Verification items for the finished model (mm, model axes). Face numbers are marked on the shaded views. Give positions to 0.01 mm unless a question says otherwise; leave off trailing zeros. Loops run counter-clockwise (first coordinate to the right, second up) from the corner with the lowest first, then second, coordinate; pieces in that order, holes last. Notation, with made-up numbers: M 42.5,81 L 47.5,81 A20 cw 47.5,96 Z; hole C 39,7 d9. An arc over 180 degrees is marked long. Put each result on its own line as item: value. Start each with the question number.
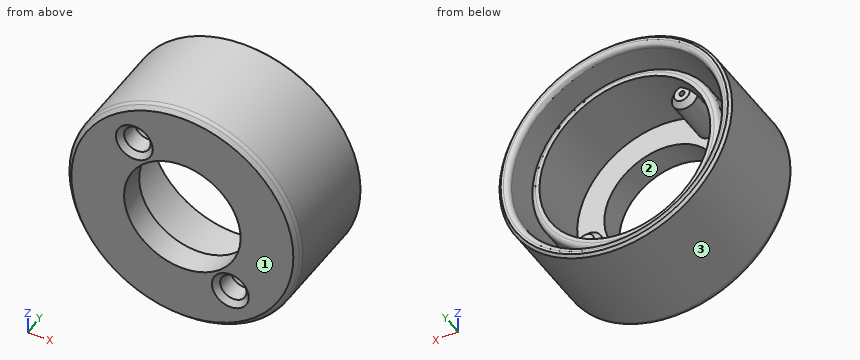
from build123d import *
from OCP.BRepFilletAPI import BRepFilletAPI_MakeChamfer

# Parameters (mm, degrees)
CROQUIS1_R              = 22.05
CROQUIS1_R_2            = 20.05
SALIENTE_EXTRUIR1_DEPTH = 16
CROQUIS1_4_R            = 17.95
CROQUIS1_4_R_2          = 16.2
SALIENTE_EXTRUIR2_DEPTH = 12.5
SALIENTE_EXTRUIR4_START = -5
CROQUIS1_6_R            = 22.05
CROQUIS1_6_R_2          = 20.05
CROQUIS1_6_R_3          = 17.95
CROQUIS1_6_R_4          = 16.2
SALIENTE_EXTRUIR4_DEPTH = 5
CORTAR_EXTRUIR1_REACH   = 39.595
CROQUIS4_R              = 11.05
CROQUIS4_R_2            = 0.5
CROQUIS5_R              = 2.5
CROQUIS5_R_2            = 0.5
CORTAR_EXTRUIR2_DEPTH   = 4.5
CROQUIS6_R              = 2.5
CROQUIS6_R_2            = 0.5
SALIENTE_EXTRUIR5_DEPTH = 10
REDONDEO2_R             = 1
CHAFL_N1_SIZE           = 1
REDONDEO3_R             = 1
CHAFL_N2_SIZE           = 0.5
CHAFL_N3_SIZE           = 2
CHAFL_N3_SIZE_2         = 1.154700538


with BuildPart() as part:
    # Croquis1 → Saliente-Extruir1 (new body)
    with BuildSketch(Plane(origin=(0, 0, 0), x_dir=(1, 0, 0), z_dir=(0, 1, 0))):
        with Locations(Location((0, 0, 0), (0, 0, 270))):
            Circle(CROQUIS1_R)
        with Locations(Location((0, 0, 0), (0, 0, 270))):
            Circle(CROQUIS1_R_2, mode=Mode.SUBTRACT)
    extrude(amount=SALIENTE_EXTRUIR1_DEPTH)



with BuildPart() as body_2:
    # Croquis1<4> → Saliente-Extruir2 (new body)
    with BuildSketch(Plane(origin=(0, 0, 0), x_dir=(1, 0, 0), z_dir=(0, 1, 0))):
        with Locations(Location((0, 0, 0), (0, 0, 270))):
            Circle(CROQUIS1_4_R)
        with Locations(Location((0, 0, 0), (0, 0, 270))):
            Circle(CROQUIS1_4_R_2, mode=Mode.SUBTRACT)
    extrude(amount=SALIENTE_EXTRUIR2_DEPTH)


with BuildPart() as part_1:
    add(part.part)

    add(body_2.part)  # Saliente-Extruir4 merges body 2
    # Croquis1<6> → Saliente-Extruir4 (add)
    # profile 1 of 4: a face of its own
    with BuildSketch(Plane(origin=(0, 0, 0), x_dir=(1, 0, 0), z_dir=(0, 1, 0)).offset(SALIENTE_EXTRUIR4_START)):
        with Locations(Location((0, 0, 0), (0, 0, 270))):
            Circle(CROQUIS1_6_R)
        with Locations(Location((0, 0, 0), (0, 0, 270))):
            Circle(CROQUIS1_6_R_2, mode=Mode.SUBTRACT)
    # profile 2 of 4: a face of its own
    with BuildSketch(Plane(origin=(0, 0, 0), x_dir=(1, 0, 0), z_dir=(0, 1, 0)).offset(SALIENTE_EXTRUIR4_START)):
        with Locations(Location((0, 0, 0), (0, 0, 270))):
            Circle(CROQUIS1_6_R_2)
        with Locations(Location((0, 0, 0), (0, 0, 270))):
            Circle(CROQUIS1_6_R_3, mode=Mode.SUBTRACT)
    # profile 3 of 4: a face of its own
    with BuildSketch(Plane(origin=(0, 0, 0), x_dir=(1, 0, 0), z_dir=(0, 1, 0)).offset(SALIENTE_EXTRUIR4_START)):
        with Locations(Location((0, 0, 0), (0, 0, 270))):
            Circle(CROQUIS1_6_R_3)
        with Locations(Location((0, 0, 0), (0, 0, 270))):
            Circle(CROQUIS1_6_R_4, mode=Mode.SUBTRACT)
    # profile 4 of 4: a face of its own
    with BuildSketch(Plane(origin=(0, 0, 0), x_dir=(1, 0, 0), z_dir=(0, 1, 0)).offset(SALIENTE_EXTRUIR4_START)):
        with Locations(Location((0, 0, 0), (0, 0, 270))):
            Circle(CROQUIS1_6_R_4)
    extrude(amount=SALIENTE_EXTRUIR4_DEPTH)

    # Croquis4 → Cortar-Extruir1 (cut, up to next)
    with BuildSketch(Plane.XZ.offset(5), mode=Mode.PRIVATE) as cortar_extruir1_sk1:
        with Locations(Location((0, 0, 0), (0, 0, 270))):
            Circle(CROQUIS4_R)
    cortar_extruir1_tool1 = extrude(cortar_extruir1_sk1.sketch, amount=-CORTAR_EXTRUIR1_REACH, mode=Mode.PRIVATE) & part_1.part
    # Croquis4 → Cortar-Extruir1 (cut, up to next)
    with BuildSketch(Plane.XZ.offset(5), mode=Mode.PRIVATE) as cortar_extruir1_sk2:
        with Locations(Location((-9.1, 12.1, 0), (0, 0, 270))):
            Circle(CROQUIS4_R_2)
    cortar_extruir1_tool2 = extrude(cortar_extruir1_sk2.sketch, amount=-CORTAR_EXTRUIR1_REACH, mode=Mode.PRIVATE) & part_1.part
    # Croquis4 → Cortar-Extruir1 (cut, up to next)
    with BuildSketch(Plane.XZ.offset(5), mode=Mode.PRIVATE) as cortar_extruir1_sk3:
        with Locations(Location((9.1, -12.1, 0), (0, 0, 270))):
            Circle(CROQUIS4_R_2)
    cortar_extruir1_tool3 = extrude(cortar_extruir1_sk3.sketch, amount=-CORTAR_EXTRUIR1_REACH, mode=Mode.PRIVATE) & part_1.part
    add(cortar_extruir1_tool1.solids().sort_by_distance((0, -5, 0))[0], mode=Mode.SUBTRACT)
    add(cortar_extruir1_tool2.solids().sort_by_distance((-9.1, -5, 12.1))[0], mode=Mode.SUBTRACT)
    add(cortar_extruir1_tool3.solids().sort_by_distance((9.1, -5, -12.1))[0], mode=Mode.SUBTRACT)

    # Croquis5 → Cortar-Extruir2 (cut)
    # profile 1 of 2: a face of its own
    with BuildSketch(Plane.XZ.offset(5)):
        with Locations(Location((-9.1, 12.1, 0), (0, 0, 270))):
            Circle(CROQUIS5_R)
        with Locations(Location((-9.1, 12.1, 0), (0, 0, 270))):
            Circle(CROQUIS5_R_2, mode=Mode.SUBTRACT)
    # profile 2 of 2: a face of its own
    with BuildSketch(Plane.XZ.offset(5)):
        with Locations(Location((9.1, -12.1, 0), (0, 0, 270))):
            Circle(CROQUIS5_R)
        with Locations(Location((9.1, -12.1, 0), (0, 0, 270))):
            Circle(CROQUIS5_R_2, mode=Mode.SUBTRACT)
    extrude(amount=-CORTAR_EXTRUIR2_DEPTH, mode=Mode.SUBTRACT)

    # Croquis6 → Saliente-Extruir5 (add)
    # profile 1 of 2: a face of its own
    with BuildSketch(Plane.XZ.offset(0.5)):
        with Locations(Location((-9.1, 12.1, 0), (0, 0, 270))):
            Circle(CROQUIS6_R)
        with Locations(Location((-9.1, 12.1, 0), (0, 0, 270))):
            Circle(CROQUIS6_R_2, mode=Mode.SUBTRACT)
    # profile 2 of 2: a face of its own
    with BuildSketch(Plane.XZ.offset(0.5)):
        with Locations(Location((9.1, -12.1, 0), (0, 0, 270))):
            Circle(CROQUIS6_R)
        with Locations(Location((9.1, -12.1, 0), (0, 0, 270))):
            Circle(CROQUIS6_R_2, mode=Mode.SUBTRACT)
    extrude(amount=-SALIENTE_EXTRUIR5_DEPTH)

    # Redondeo2
    redondeo2_edges = [part_1.edges().sort_by_distance(p)[0] for p in [
        (0, 12.5, -17.95),
        (0, 16, -20.05),
    ]]
    fillet(redondeo2_edges, radius=REDONDEO2_R)

    # Chaflán1
    chafl_n1_edges = [part_1.edges().sort_by_distance(p)[0] for p in [
        (-9.1, -5, 14.6),
        (9.1, -5, -9.6),
        (-7.597359303, 9.5, 10.101983249),
        (7.597359303, 9.5, -10.101983249),
        (0, -5, -22.05),
    ]]
    chamfer(chafl_n1_edges, length=CHAFL_N1_SIZE)

    # Redondeo3
    redondeo3_edges = [part_1.edges().sort_by_distance(p)[0] for p in [
        (0, -4, -22.05),
    ]]
    fillet(redondeo3_edges, radius=REDONDEO3_R)

    # Chaflán2
    chafl_n2_edges = [part_1.edges().sort_by_distance(p)[0] for p in [
        (0, 16, -22.05),
    ]]
    chamfer(chafl_n2_edges, length=CHAFL_N2_SIZE)

    # Chaflán3
    chafl_n3_edges_1 = [part_1.edges().sort_by_distance(p)[0] for p in [
        (-9.1, -0.5, 12.6),
    ]]
    chafl_n3_side_1 = [part_1.faces().sort_by_distance(p)[0] for p in [
        (-9.1, -0.5, 12.623094011),
    ]]
    chafl_n3_edges_2 = [part_1.edges().sort_by_distance(p)[0] for p in [
        (9.1, -0.5, -11.6),
    ]]
    chafl_n3_side_2 = [part_1.faces().sort_by_distance(p)[0] for p in [
        (9.1, -0.5, -11.576905989),
    ]]
    chafl_n3 = BRepFilletAPI_MakeChamfer(part_1.part.solid().wrapped)
    for e in chafl_n3_edges_1:
        chafl_n3.Add(CHAFL_N3_SIZE - 0.0001, CHAFL_N3_SIZE_2 - 0.0001, e.wrapped, chafl_n3_side_1[0].wrapped)
    for e in chafl_n3_edges_2:
        chafl_n3.Add(CHAFL_N3_SIZE - 0.0001, CHAFL_N3_SIZE_2 - 0.0001, e.wrapped, chafl_n3_side_2[0].wrapped)
    add(Compound.cast(chafl_n3.Shape()), mode=Mode.REPLACE)  # a hair under: the kernel refuses the full size


solid = part_1.part
Q1. Release check for a two-part mould opening along Z. For the marked faces 1, 2 and 3 record: pulls with the +Z half, pulls with the -Z half, needs draft (parallel to the pull), parting line crosses it, or undercut.
Q2. Go/stop test with flat-tipped pins: pin 1 (6 mm diameter, centred on x = -9.1, z = 12.1, fed in from +Y); pin 2 (10 mm diameter, centred on y = 7.5, z = 12.5, fed in from -X); pin 3 (3 mm diameter, centred on x = 15.5, y = -1, fed in from +Z). Record where each tip stops, or that it passes through.
Q3. Scan lines: L1, parallel to X at y = 7.25, z = 0; L2, parallel to X at y = 2.75, z = 7; L3, parallel to Y at x = -16, z = -9. Record each from-to range of solid material in increasing order.
Q4. Cross-section at A-A, the plane y = 6.25. Record the boundary of the cut face in (x, z).
Ans:
1. face 1: needs draft
1. face 2: undercut
1. face 3: parting line crosses it
2. pin 1: stops at y = 12.5
2. pin 2: stops at x = -20.74
2. pin 3: stops at z = 17.04
3. L1: x = -22.05 to -20.05, -17.95 to -16.2, 16.2 to 17.95, 20.05 to 22.05
3. L2: x = -20.91 to -18.79, -16.53 to -14.61, 14.61 to 16.53, 18.79 to 20.91
3. L3: y = -5 to 0
4. outline: C 0,0 d44.1; C 0,0 d35.9; hole C 0,0 d40.1; hole M -11.5,11.41 A16.2 ccw 7.77,-14.22 A2.5 cw long 11.5,-11.41 A16.2 ccw -7.77,14.22 A2.5 cw long Z; hole C -9.1,12.1 d1; hole C 9.1,-12.1 d1
